Here's how the part is built. I have some questions about the finished solid (model axes, mm). A direction names the side the tool comes from. Round coordinates to 2 decimals unless told otherwise and drop trailing zeros. Loops run counter-clockwise (first coordinate to the right, second up) from the corner with the lowest first, then second, coordinate; pieces in that order, holes last. Notation, with made-up numbers: M 33,39 L 41,39 A29 ccw 41,61 Z; hole C 55.25,21 d10. An arc over 180 degrees is marked long. Use a Markdown table: item, result.
from build123d import *

# Parameters (mm, degrees)
F0_W     = 38
F0_H     = 8.4
F1_DEPTH = 3
F2_W     = 2.8
F2_H     = 3
F3_DEPTH = 2.8
F4_W     = 32.4
F4_H     = 3.3850746269
F5_DEPTH = 25


# Not quite as in the source:
# - a pattern or mirror of a feature is missing from the dataset's text; its kind, count and spacing are read off the source's solid


with BuildPart() as f1:
    # F0 (on Top) → F1 (new body)
    with BuildSketch(Plane.XY):
        Rectangle(F0_W, F0_H)
    extrude(amount=F1_DEPTH)

    # F2 (on face) → F3 (join)
    with BuildSketch(Plane(origin=(-19, 0, 0), x_dir=(0, -1, 0), z_dir=(-1, 0, 0))):
        with Locations((-2.8, 1.5)):
            Rectangle(F2_W, F2_H)
        with Locations((2.8, 1.5)):
            Rectangle(F2_W, F2_H)
    f3 = extrude(amount=F3_DEPTH)

    # F3_copies: F3 across plane
    add(f3.mirror(Plane(origin=(0, 0, 0), x_dir=(0, 0, 1), z_dir=(1, 0, 0))))

    # F4 (on face) → F5 (cut)
    with BuildSketch(Plane.XY.offset(3)):
        Rectangle(F4_W, F4_H)
    extrude(amount=-F5_DEPTH, mode=Mode.SUBTRACT)


solid = f1.part
1. Imagine slicing it at A-A, the plane y = 0. Write out the boundary of the cut face in (x, z).
Answer sheet:
| item | result |
|---|---|
| outline | M -19,0 L -16.2,0 L -16.2,3 L -19,3 Z; M 16.2,0 L 19,0 L 19,3 L 16.2,3 Z |
2. For pin 1 Ø0.8 at (y, z) = (0.5, 1.5) entering from +X; pin 2 Ø1.4 at (y, z) = (0, 1) entering from -X, each with a flat end and sliding along its axis, tell me the tip position at first contact or that it passes through.
Answer sheet:
| item | result |
|---|---|
| pin 1 | x = 19 |
| pin 2 | x = -19 |
3. Imagine slicing it at C-C, the plane z = 0.5. Write out the boundary of the cut face in (x, y).
Answer sheet:
| item | result |
|---|---|
| outline | M -21.8,-4.2 L 21.8,-4.2 L 21.8,-1.4 L 19,-1.4 L 19,1.4 L 21.8,1.4 L 21.8,4.2 L -21.8,4.2 L -21.8,1.4 L -19,1.4 L -19,-1.4 L -21.8,-1.4 Z; hole M -16.2,-1.69 L 16.2,-1.69 L 16.2,1.69 L -16.2,1.69 Z |
4. Imagine slicing it at B-B, the plane x = -12.5. Write out the boundary of the cut face in (y, z), then the cut area to 3 significant figures.
Answer sheet:
| item | result |
|---|---|
| outline | M -4.2,0 L -1.69,0 L -1.69,3 L -4.2,3 Z; M 1.69,0 L 4.2,0 L 4.2,3 L 1.69,3 Z |
| area | 15.0 mm2 |
5. Which directions (+Z, -Z, +X, -X, +Y, -Y) give clear straight access to the entire face, cutting with the end or side of a thin tool? Please do faces 1 (the face through (19, 0, 1)), 2 (the face through (0, 4.2, 1)), 3 (the face through (-20, 1.4, 1)), 4 (the face through (16.2, 0, 2)), 5 (the face through (-21.8, 3, 2)).
Answer sheet:
| item | result |
|---|---|
| face 1 | +Z, -Z, +X |
| face 2 | +Z, -Z, +X, -X, +Y |
| face 3 | +Z, -Z, -X |
| face 4 | +Z, -Z |
| face 5 | +Z, -Z, -X, +Y, -Y |
6. I need wall thicknesses on probe 1 along X at (y, z) = (-1.5, 0.7); probe 2 along Y at (x, z) = (14, 0.7); probe 3 along X at (y, z) = (-1, 2.15). Which ranges of each line are inside material? Lowest first, please. Write a range as from..to.
Answer sheet:
| item | result |
|---|---|
| probe 1 | -21.8..-16.2, 16.2..21.8 |
| probe 2 | -4.2..-1.69, 1.69..4.2 |
| probe 3 | -19..-16.2, 16.2..19 |
